The drawing under review shows one solid part. Ordinate dimensions are in mm from its lowest x, y, z. A direction names the side the tool comes from. Give positions to 0.01 mm unless a question says otherwise; leave off trailing zeros. Write each loop counter-clockwise with the first axis right and the second up, starting at its lowest first coordinate (ties: lowest second). Pieces come first, ordered by that corner, then holes. Notation, with made-up numbers: (-3.75, 23.5) -> (46.25, 23.5) arc R14 cw to (46.25, 27.5) -> close; hole circle Ø7 at (66.5, -14). An arc over 180 degrees is marked (long way). Answer as a JSON object with one key per item and string values.
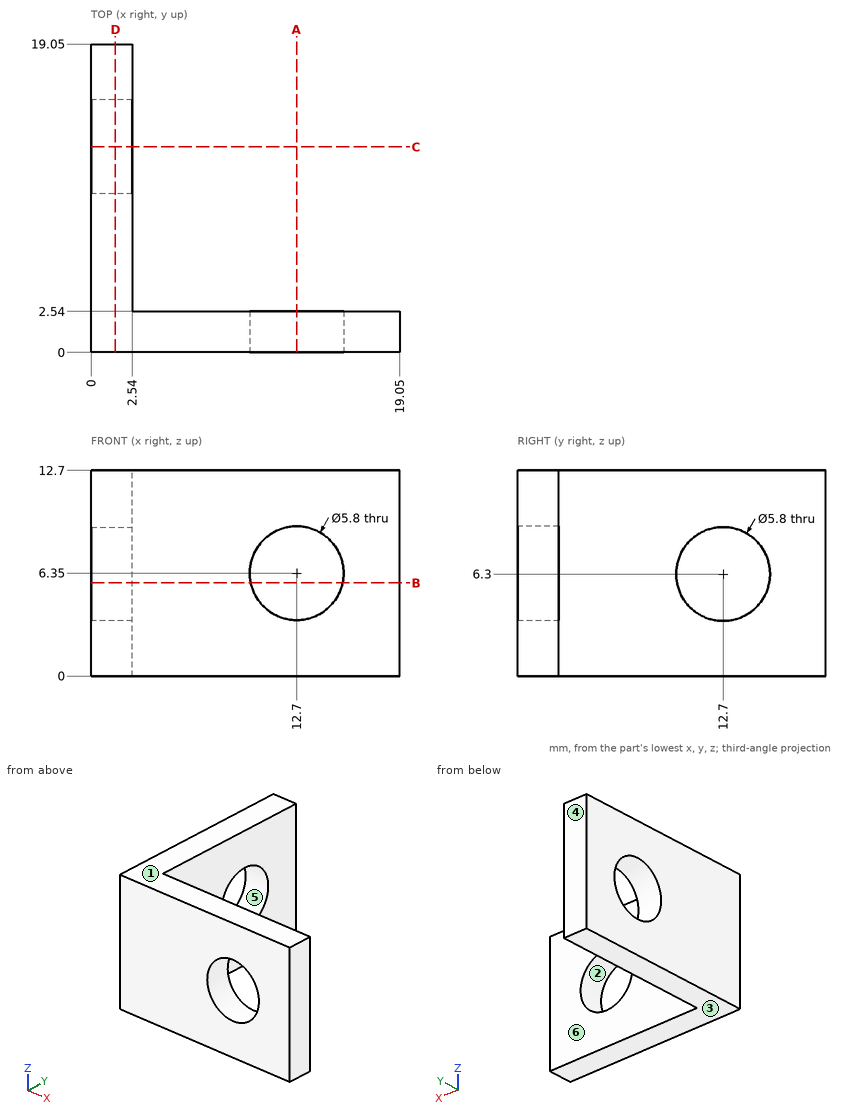
(1) We need section B-B, the plane z = 5.75. State the section outline as (x, y) points.
Here are the results:
{"outline": "(0, 0) -> (9.86, 0) -> (9.86, 2.54) -> (2.54, 2.54) -> (2.54, 9.85) -> (0, 9.85) -> close; (0, 15.55) -> (2.54, 15.55) -> (2.54, 19.05) -> (0, 19.05) -> close; (15.54, 0) -> (19.05, 0) -> (19.05, 2.54) -> (15.54, 2.54) -> close"}
(2) Clearance check with flat-ended pins moving along their axes: pin 1 (7.5 mm diameter, centred on y = 12.7, z = 6.3, fed in from +X); pin 2 (1 mm diameter, centred on x = 4.5, y = 13, fed in from +Z); pin 3 (6 mm diameter, centred on x = 14.5, z = 10.5, fed in from +Y). State where each tip first meets the part, or that it passes through.
Here are the results:
{"pin 1": "stops at x = 2.54", "pin 2": "passes through", "pin 3": "stops at y = 2.54"}
(3) We need section C-C, the plane y = 12.7. State the section outline as (x, z) points.
Here are the results:
{"outline": "(0, 0) -> (2.54, 0) -> (2.54, 3.4) -> (0, 3.4) -> close; (0, 9.2) -> (2.54, 9.2) -> (2.54, 12.7) -> (0, 12.7) -> close"}
(4) For the marked faces 5 and 6, list the 3-axis set-ups (+Z, -Z, +X, -X, +Y, -Y) from which the entire face can be reached by the end or side of a thin tool; tool diameter is ignored.
Here are the results:
{"face 5": "+X, -X", "face 6": "+Z, -Z, +X, +Y"}
(5) For line 1 along X through (y, z) = (1.55, 6.35); line 2 along Z through (x, y) = (12.7, 1.55); line 3 along Z through (x, y) = (0.65, 12.7), list the stretches that pass through material, from the lowest coordinate up.
Here are the results:
{"line 1": "x = 0 to 9.8, 15.6 to 19.05", "line 2": "z = 0 to 3.45, 9.25 to 12.7", "line 3": "z = 0 to 3.4, 9.2 to 12.7"}
(6) We need section A-A, the plane x = 12.7. State the section outline as (y, z) points.
Here are the results:
{"outline": "(0, 0) -> (2.54, 0) -> (2.54, 3.45) -> (0, 3.45) -> close; (0, 9.25) -> (2.54, 9.25) -> (2.54, 12.7) -> (0, 12.7) -> close"}
(7) The part is to be moulded in two halves that separate along Z. For the marked faces 1, 2, 3 and 4, say which applies: +Z half, -Z half, draft (parallel to the pull), parting line (faces both ways), or undercut.
Here are the results:
{"face 1": "+Z half", "face 2": "undercut", "face 3": "-Z half", "face 4": "draft"}
(8) We need section D-D, the plane x = 1.5. State the section outline as (y, z) points, then the cut area to 4 significant figures.
Here are the results:
{"outline": "(0, 0) -> (19.05, 0) -> (19.05, 12.7) -> (0, 12.7) -> close; hole circle Ø5.8 at (12.7, 6.3)", "area": "215.5 mm²"}
